Part print with two shaded views. Sizes in mm from the minimum x, y, z corner. Round coordinates to 2 decimals unless told otherwise and drop trailing zeros. Write each loop counter-clockwise with the first axis right and the second up, starting at its lowest first coordinate (ties: lowest second). Pieces come first, ordered by that corner, then holes. Notation, with made-up numbers: (33.25, -39.75) -> (72.25, -39.75) arc R6 cw to (72.25, -29.75) -> close; hole circle Ø2 at (25.25, 62). An arc over 180 degrees is marked (long way). Answer in a Markdown table with one row per item. Add a question column.
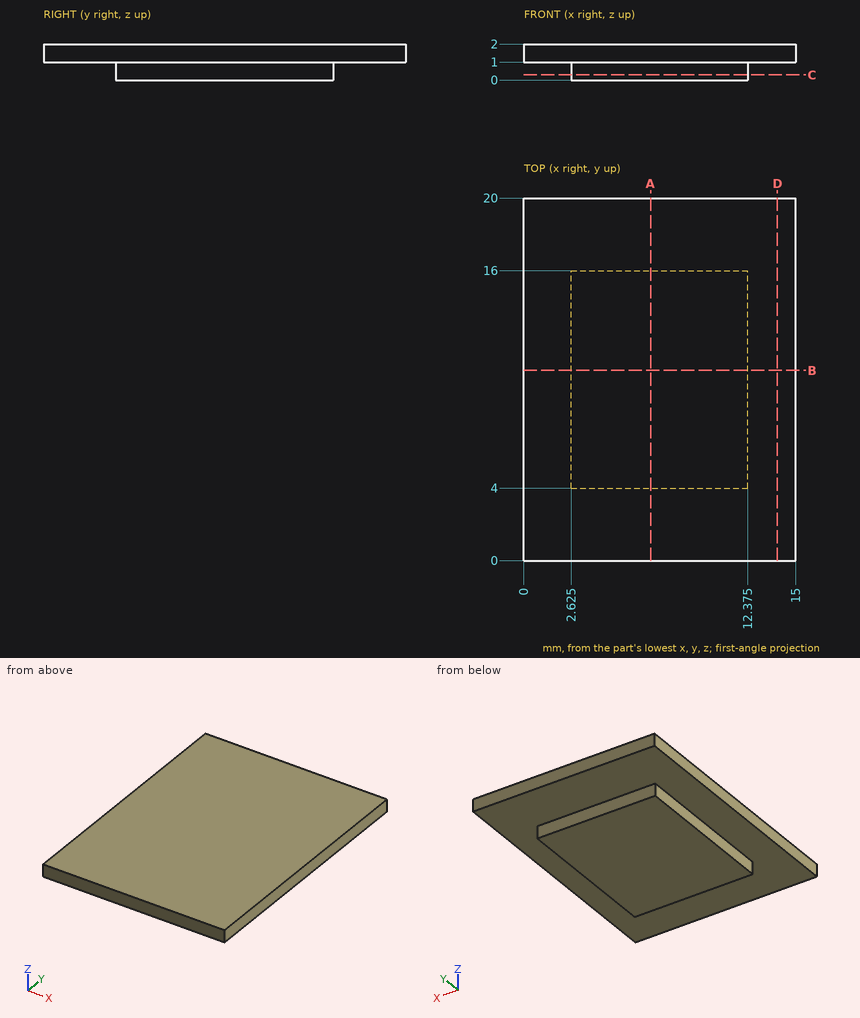
Item 1: Drill centre lines: probe 1 along Z at (x, y) = (5.5, 3.25); probe 2 along Y at (x, z) = (3, 0.75); probe 3 along X at (y, z) = (15.75, 0.9) (3 decimals). Where is each one in solid material? Low to high.
Item 2: Saw through at C-C on z = 0.3. Give the cut face in (x, y) (3 decimals), then the cut area to 3 significant figures.
Item 3: Saw through at A-A on x = 7. Give the cut face in (y, z), then the cut area to 3 significant figures.
Item 4: Pin check, flat tips, straight feed: pin 1 (5 mm diameter, centred on x = 5, y = 5.5, fed in from -Z); pin 2 (0.5 mm diameter, centred on x = 8.5, z = 0.5, fed in from +Y); pin 3 (0.8 mm diameter, centred on x = 9.5, z = 0.5, fed in from -Y); pin 4 (0.8 mm diameter, centred on y = 11, z = 0.5, fed in from +X) (3 decimals). Stop position of each tip, or through.
Item 5: Saw through at B-B on y = 10.5. Give the cut face in (x, z) (3 decimals), then the cut area to 4 significant figures.
Item 6: Saw through at D-D on x = 14. Give the cut face in (y, z).
Recorded:
| question | item | result |
|---|---|---|
| 1 | probe 1 | 1 to 2 |
| 1 | probe 2 | 4 to 16 |
| 1 | probe 3 | 2.625 to 12.375 |
| 2 | outline | (2.625, 4) -> (12.375, 4) -> (12.375, 16) -> (2.625, 16) -> close |
| 2 | area | 117 mm2 |
| 3 | outline | (0, 1) -> (4, 1) -> (4, 0) -> (16, 0) -> (16, 1) -> (20, 1) -> (20, 2) -> (0, 2) -> close |
| 3 | area | 32.0 mm2 |
| 4 | pin 1 | z = 0 |
| 4 | pin 2 | y = 16 |
| 4 | pin 3 | y = 4 |
| 4 | pin 4 | x = 12.375 |
| 5 | outline | (0, 1) -> (2.625, 1) -> (2.625, 0) -> (12.375, 0) -> (12.375, 1) -> (15, 1) -> (15, 2) -> (0, 2) -> close |
| 5 | area | 24.75 mm2 |
| 6 | outline | (0, 1) -> (20, 1) -> (20, 2) -> (0, 2) -> close |
